Could you check a few things on this model? Use its own coordinates, in mm. A direction names the side the tool comes from. Give positions to 0.01 mm unless a question says otherwise; leave off trailing zeros. Loops run counter-clockwise (first coordinate to the right, second up) from the corner with the lowest first, then second, coordinate; pieces in that order, holes last. Notation, with made-up numbers: M 19.25,2.5 L 64.25,2.5 A23 cw 64.25,40.5 Z; hole C 86.5,73 d10. An arc over 180 degrees is marked long. Answer in a Markdown table with one row per item. Add a question column.
1. I need wall thicknesses on line 1 along Z through (x, y) = (19.5, -8.5); line 2 along Z through (x, y) = (20.5, -3.5); line 3 along X through (y, z) = (-11, 6). Which ranges of each line are inside material? Lowest first, please. Write a range as from..to.
2. If we section it at C-C on x = -28.75: List the corners of the cut face in (y, z) for me.
3. If we section it at A-A on y = -11: List the corners of the cut face in (x, z) for me.
4. I'm going to push flat-ended pins straight in: pin 1 Ø1.5 at (y, z) = (3, -22) entering from -X; pin 2 Ø6.5 at (x, z) = (39.5, 23) entering from -Y; pin 3 Ø4 at (y, z) = (-2.5, 21) entering from +X; pin 4 Ø2.5 at (y, z) = (6.5, -32) entering from +X. Where does each tip first touch, or does it pass through?
5. Which directions (+Z, -Z, +X, -X, +Y, -Y) give clear straight access to the entire face, cutting with the end or side of a thin tool? Please do faces 4 (the flat face through (24, -10, -32)), 5 (the cylindrical face through (-32.97, -10.35, 11.89)), 6 (the flat face through (37.25, -4, 21)), 7 (the flat face through (45.25, -4, 21)), 8 (the flat face through (41, -4, 5.5)).
6. If we section it at D-D on z = -20: List the corners of the cut face in (x, y) for me.
7. If we section it at B-B on z = 3.5: List the corners of the cut face in (x, y) for me, then the cut area to 3 significant figures.
8. Thinking about a two-plate mould opening in X: for faces 1 (the flat face through (44.111, 4.951, -34.814)), 2 (the flat face through (40.065, 5, 31)), 3 (the flat face through (41, -7.5, 10)), which applies, released by +X, released by -X, zero draft, split by the parting line, or undercut?
```python
from build123d import *

# Parameters (mm, degrees)
SKETCH_1_W       = 93.5
SKETCH_1_H       = 73
EXTRUDE_1_DEPTH  = 1.5
CHAMFER_1_SIZE   = 1
EXTRUDE_2_DEPTH  = 7
SKETCH_3_W       = 30
SKETCH_3_H       = 30
EXTRUDE_3_DEPTH  = 24
SKETCH_4_R       = 6.25
EXTRUDE_4_DEPTH  = 21
SKETCH_5_R       = 6.25
EXTRUDE_5_DEPTH  = 21
SKETCH_6_R       = 6.25
EXTRUDE_6_DEPTH  = 21
SKETCH_8_W       = 8
SKETCH_8_H       = 8
EXTRUDE_7_DEPTH  = 7.5
SKETCH_9_R       = 6.5
EXTRUDE_9_DEPTH  = 20.5
SKETCH_10_W      = 22.5
SKETCH_10_H      = 5.6
EXTRUDE_10_DEPTH = 10


with BuildPart() as part:
    # Эскиз1 → Бобышка-Вытянуть1 (new body)
    with BuildSketch(Plane(origin=(0, 0, 0), x_dir=(1, 0, 0), z_dir=(0, 1, 0))):
        Rectangle(SKETCH_1_W, SKETCH_1_H)
    extrude(amount=EXTRUDE_1_DEPTH)

    # Фаска1
    chamfer_1_edges = [part.edges().sort_by_distance(p)[0] for p in [
        (46.75, 0.75, 36.5),
        (-46.75, 0.75, 36.5),
        (-46.75, 0.75, -36.5),
        (46.75, 0.75, -36.5),
    ]]
    chamfer(chamfer_1_edges, length=CHAMFER_1_SIZE)

    # Эскиз2 → Бобышка-Вытянуть2 (add)
    with BuildSketch(Plane(origin=(0, 1.5, 0), x_dir=(1, 0, 0), z_dir=(0, 1, 0))):
        Polygon((42.75, 35.6), (40.065321248, 34.05), (40.065321248, 30.95), (42.75, 29.4), (45.434678752, 30.95), (45.434678752, 34.05), align=None)
        Polygon((-43.25, 35.6), (-45.934678752, 34.05), (-45.934678752, 30.95), (-43.25, 29.4), (-40.565321248, 30.95), (-40.565321248, 34.05), align=None)
        Polygon((42.75, -28.4), (40.065321248, -29.95), (40.065321248, -33.05), (42.75, -34.6), (45.434678752, -33.05), (45.434678752, -29.95), align=None)
        Polygon((-43.25, -28.4), (-45.934678752, -29.95), (-45.934678752, -33.05), (-43.25, -34.6), (-40.565321248, -33.05), (-40.565321248, -29.95), align=None)
    extrude(amount=EXTRUDE_2_DEPTH)

    # Эскиз3 → Бобышка-Вытянуть3 (add)
    with BuildSketch(Plane.XZ):
        with Locations((-2.75, 20)):
            Rectangle(SKETCH_3_W, SKETCH_3_H)
    extrude(amount=EXTRUDE_3_DEPTH)

    # Эскиз4 → Бобышка-Вытянуть4 (add)
    with BuildSketch(Plane.XZ):
        with Locations(Location((-31.25, 29.5, 0), (0, 0, 90))):
            Circle(SKETCH_4_R)
    extrude(amount=EXTRUDE_4_DEPTH)

    # Эскиз5 → Бобышка-Вытянуть5 (add)
    with BuildSketch(Plane.XZ):
        with Locations(Location((-28.75, 16.5, 0), (0, 0, 90))):
            Circle(SKETCH_5_R)
    extrude(amount=EXTRUDE_5_DEPTH)

    # Эскиз6 → Бобышка-Вытянуть6 (add)
    with BuildSketch(Plane.XZ):
        with Locations(Location((-30.75, 3.5, 0), (0, 0, 90))):
            Circle(SKETCH_6_R)
    extrude(amount=EXTRUDE_6_DEPTH)

    # Эскиз8 → Бобышка-Вытянуть7 (add)
    with BuildSketch(Plane.XZ):
        with Locations((-41.25, 21.5)):
            Rectangle(SKETCH_8_W, SKETCH_8_H)
        with Locations((-41.25, 9.5)):
            Rectangle(SKETCH_8_W, SKETCH_8_H)
        with Locations((41.25, 21.5)):
            Rectangle(SKETCH_8_W, SKETCH_8_H)
        with Locations((41.25, 9.5)):
            Rectangle(SKETCH_8_W, SKETCH_8_H)
    extrude(amount=EXTRUDE_7_DEPTH)

    # Эскиз9 → Бобышка-Вытянуть9 (add)
    with BuildSketch(Plane.XZ):
        with Locations(Location((16.917714538, -5.160483157, 0), (0, 0, 90))):
            Circle(SKETCH_9_R)
        with Locations(Location((24.917714538, -16.160483157, 0), (0, 0, 90))):
            Circle(SKETCH_9_R)
    extrude(amount=EXTRUDE_9_DEPTH)

    # Эскиз10 → Бобышка-Вытянуть10 (add)
    with BuildSketch(Plane.XZ):
        with Locations((-23.9, -32.107649626)):
            Rectangle(SKETCH_10_W, SKETCH_10_H)
        with Locations((24.6, -32.107649626)):
            Rectangle(SKETCH_10_W, SKETCH_10_H)
    extrude(amount=EXTRUDE_10_DEPTH)


solid = part.part
```
Results:
| question | item | result |
|---|---|---|
| 1 | line 1 | -34.91..-29.31, -19.75..-12.57, -11.13..0.8 |
| 1 | line 2 | -34.91..-29.31, -20.93..-11.39, -10.58..0.26 |
| 1 | line 3 | -36.48..-25.02, -17.75..12.25 |
| 2 | outline | M -21,-2.42 L 0,-2.42 L 0,-29.31 L -10,-29.31 L -10,-34.91 L 0,-34.91 L 0,-36.5 L 1.5,-36.5 L 1.5,36.5 L 0,36.5 L 0,35.23 L -21,35.23 L -21,23.77 L 0,23.77 L 0,22.75 L -21,22.75 L -21,10.25 L 0,10.25 L 0,9.42 L -21,9.42 Z |
| 3 | outline | C -31.25,29.5 d12.5; C -30.75,3.5 d12.5; C -28.75,16.5 d12.5; M -17.75,5 L 12.25,5 L 12.25,35 L -17.75,35 Z; C 16.92,-5.16 d13; C 24.92,-16.16 d13 |
| 4 | pin 1 | through |
| 4 | pin 2 | y = -7.5 |
| 4 | pin 3 | x = 45.25 |
| 4 | pin 4 | x = 45.43 |
| 5 | face 4 | -Z, +X, -X, -Y |
| 5 | face 5 | -Y |
| 5 | face 6 | +Z, -Z, -Y |
| 5 | face 7 | +Z, -Z, +X, -Y |
| 5 | face 8 | -Z, +X, -Y |
| 6 | outline | M -46.75,0 L 19.67,0 L 19.67,-20.5 L 30.16,-20.5 L 30.16,0 L 46.75,0 L 46.75,1.5 L -46.75,1.5 Z |
| 7 | outline | M -46.75,0 L -37,0 L -37,-21 L -24.5,-21 L -24.5,0 L 46.75,0 L 46.75,1.5 L -46.75,1.5 Z |
| 7 | area | 403 mm2 |
| 8 | face 1 | released by +X |
| 8 | face 2 | undercut |
| 8 | face 3 | zero draft |
